from build123d import *

# Parameters (mm, degrees)
SKETCH1_R                = 23.72487
BOSS_EXTRUDE1_DEPTH      = 31.75
SKETCH2_W                = 47.44974
SKETCH2_H                = 6.35
BOSS_EXTRUDE2_DEPTH      = 25.4
SKETCH3_W                = 12.7
SKETCH3_H                = 68.28282
BOSS_EXTRUDE3_DEPTH      = 13.65758
SKETCH4_W                = 12.7
SKETCH4_H                = 2.43586
BOSS_EXTRUDE4_DEPTH      = 38.0746
SKETCH5_W                = 12.7
SKETCH5_H                = 27.81554
SKETCH5_H_2              = 30.2514
BOSS_EXTRUDE5_DEPTH      = 0.70358
BOSS_EXTRUDE8_REACH      = 72.166
BOSS_EXTRUDE8_END_RADIUS = 23.72487
SKETCH9_W                = 2.54
SKETCH9_H                = 47.44974


with BuildPart() as part:
    # Sketch1 → Boss-Extrude1 (new body)
    with BuildSketch(Plane.YZ):
        with Locations(Location((0, 0, 0), (0, 0, 270))):
            Circle(SKETCH1_R)
    extrude(amount=BOSS_EXTRUDE1_DEPTH)

    # Sketch2 → Boss-Extrude2 (add)
    with BuildSketch(Plane(origin=(0, 0, 0), x_dir=(0, 1, 0), z_dir=(0, 0, 1))):
        with Locations((0, -3.175)):
            Rectangle(SKETCH2_W, SKETCH2_H)
    extrude(amount=BOSS_EXTRUDE2_DEPTH)

    # Sketch3 → Boss-Extrude3 (add)
    with BuildSketch(Plane.XY.offset(25.4)):
        with Locations((6.35, 0)):
            Rectangle(SKETCH3_W, SKETCH3_H)
    extrude(amount=BOSS_EXTRUDE3_DEPTH)

    # Sketch4 → Boss-Extrude4 (add)
    with BuildSketch(Plane.XY.offset(39.05758)):
        with Locations((6.35, 32.92348)):
            Rectangle(SKETCH4_W, SKETCH4_H)
        with Locations((6.35, -32.92348)):
            Rectangle(SKETCH4_W, SKETCH4_H)
    extrude(amount=BOSS_EXTRUDE4_DEPTH)

    # Sketch5 → Boss-Extrude5 (add)
    with BuildSketch(Plane.XY.offset(77.13218)):
        with Locations((6.35, 20.23364)):
            Rectangle(SKETCH5_W, SKETCH5_H)
        with Locations((6.35, -19.01571)):
            Rectangle(SKETCH5_W, SKETCH5_H_2)
    extrude(amount=BOSS_EXTRUDE5_DEPTH)

    # Boss-Extrude8: up to this cylinder (the profile starts outside it)
    boss_extrude8_end = Plane(origin=(11.43, 0, 0), z_dir=(-1, 0, 0)) * Cylinder(BOSS_EXTRUDE8_END_RADIUS, 192.78174, mode=Mode.PRIVATE)
    # Sketch9 → Boss-Extrude8 (add, up to the surface)
    with BuildSketch(Plane(origin=(0, 0, 25.4), x_dir=(1, 0, 0), z_dir=(0, 0, -1)), mode=Mode.PRIVATE) as boss_extrude8_sk1:
        with Locations((11.43, 0)):
            Rectangle(SKETCH9_W, SKETCH9_H)
    boss_extrude8_tool1 = extrude(boss_extrude8_sk1.sketch, amount=BOSS_EXTRUDE8_REACH, mode=Mode.PRIVATE) - boss_extrude8_end
    add(boss_extrude8_tool1.solids().sort_by_distance((11.43, 0, 25.4))[0])


solid = part.part
Read the model definition and answer for the solid it produces. Units are mm, in the model's axes. A direction names the side the tool comes from. Round coordinates to 2 decimals unless told otherwise and drop trailing zeros. Order: outer loops, then holes, each group sorted by start corner. A loop starts at its lowest first (then second) coordinate and runs counter-clockwise, first axis right, second up.
1) The part is cut by section B-B on x = 9. Write down the section's boundary in (y, z), plus the area to 3 significant figures.
2) The part is cut by section C-C on z = 68.5. Write down the section's boundary in (x, y), plus the area to 3 significant figures.
3) Straight lines are drawn through the part: L1, parallel to X at y = 17.5, z = 25; L2, parallel to Z at x = 12.5, y = -28; L3, parallel to Y at x = 12, z = 56. For each, find the intervals that lie inside material, in ascending order.
4) The part is cut by section A-A on y = -26. Write down the section's boundary in (x, z).
5) The part is cut by section D-D on y = -6. Write down the section's boundary in (x, z).
6) The mould has two halves that part along Z. Classify faces 1 (the face through (6, -19, 77.836)), 2 (the face through (11, -23.725, 13)), 3 (the face through (6, -31.706, 58)): released by +Z, released by -Z, zero draft, split by the parting line, or undercut.
7) Flat-ended cylindrical pins translate along their axes: pin 1 (12 mm diameter, centred on y = 0.5, z = 31.5, fed in from +X); pin 2 (4 mm diameter, centred on x = 24.5, y = -1.5, fed in from +Z); pin 3 (4 mm diameter, centred on x = 4, y = -23.5, fed in from -Z); pin 4 (4 mm diameter, centred on x = 22.5, y = -26.5, fed in from -Z). Find the tip coordinate at first contact, or state that the pin passes through.
8) For faces 4 (the face through (11, 23.725, 13)), 5 (the face through (6, 31.706, 58)), 6 (the face through (6.35, 0, 25)), 7 (the face through (0, 0, 15)), 8 (the face through (6, 34.141, 51)), determine the directions among +Z, -Z, +X, -X, +Y, -Y from which every point of the face is accessible in a straight line to the end or side of a thin tool.
Resolved:
1. outline: (-34.14, 25.4) - (34.14, 25.4) - (34.14, 77.84) - (6.33, 77.84) - (6.33, 77.13) - (31.71, 77.13) - (31.71, 39.06) - (-31.71, 39.06) - (-31.71, 77.13) - (-3.89, 77.13) - (-3.89, 77.84) - (-34.14, 77.84) - close; circle Ø47.45 at (0, 0)
1. area: 2,930 mm2
2. outline: (0, -34.14) - (12.7, -34.14) - (12.7, -31.71) - (0, -31.71) - close; (0, 31.71) - (12.7, 31.71) - (12.7, 34.14) - (0, 34.14) - close
2. area: 61.9 mm2
3. L1: x = 0 to 6.35, 10.16 to 12.7
3. L2: z = 25.4 to 39.06, 77.13 to 77.84
3. L3: y = -34.14 to -31.71, 31.71 to 34.14
4. outline: (0, 25.4) - (12.7, 25.4) - (12.7, 39.06) - (0, 39.06) - close; (0, 77.13) - (12.7, 77.13) - (12.7, 77.84) - (0, 77.84) - close
5. outline: (0, -22.95) - (31.75, -22.95) - (31.75, 22.95) - (12.7, 22.95) - (12.7, 39.06) - (0, 39.06) - close; (0, 77.13) - (12.7, 77.13) - (12.7, 77.84) - (0, 77.84) - close; hole (6.35, 22.95) - (10.16, 22.95) - (10.16, 25.4) - (6.35, 25.4) - close
6. face 1: released by +Z
6. face 2: zero draft
6. face 3: undercut
7. pin 1: stops at x = 12.7
7. pin 2: stops at z = 23.72
7. pin 3: stops at z = -10.03
7. pin 4: passes through
8. face 4: -Z, +X, -X, +Y
8. face 5: +X, -X
8. face 6: none
8. face 7: +Z, -Z, -X, +Y, -Y
8. face 8: +Z, -Z, +X, -X, +Y
